from build123d import *

# Parameters (mm, degrees)
F1_DEPTH = 70
F3_DEPTH = 5
F4_DEPTH = 25


with BuildPart() as f1:
    # F0 (on Front) → F1 (new body)
    with BuildSketch(Plane.XZ):
        Polygon((-54.826997, 51.085521), (-62.88556, 51.085521), (-62.88556, -34.104981), (92.241742, -34.104981), (92.241742, -22.304947), (17.98786, -22.304947), (17.98786, 51.085521), (7.051241, 51.085521), (-13.095161, 5.612212), (-13.095161, -5.612212), (-22.592751, -5.612212), (-22.592751, 5.612212), align=None)
    extrude(amount=F1_DEPTH)

    # F2 (on face) → F3 (join)
    with BuildSketch(Plane.XY.offset(-22.304947)):
        with BuildLine():
            Line((77.980134, -20.254048), (34.15819, -20.254048))
            ThreePointArc((34.15819, -20.254048), (30.622656, -21.718514), (29.15819, -25.254048))
            Line((29.15819, -25.254048), (29.15819, -43.014842))
            ThreePointArc((29.15819, -43.014842), (30.622656, -46.550376), (34.15819, -48.014842))
            Line((34.15819, -48.014842), (77.980134, -48.014842))
            ThreePointArc((77.980134, -48.014842), (81.515667, -46.550376), (82.980134, -43.014842))
            Line((82.980134, -43.014842), (82.980134, -25.254048))
            ThreePointArc((82.980134, -25.254048), (81.515667, -21.718514), (77.980134, -20.254048))
        make_face()
        with BuildLine():
            ThreePointArc((31.707652, -28.936601), (33.172118, -25.401067), (36.707652, -23.936601))
            Line((36.707652, -23.936601), (70.1474, -23.936601))
            ThreePointArc((70.1474, -23.936601), (73.682934, -25.401067), (75.1474, -28.936601))
            Line((75.1474, -28.936601), (75.1474, -38.765739))
            ThreePointArc((75.1474, -38.765739), (73.682934, -42.301273), (70.1474, -43.765739))
            Line((70.1474, -43.765739), (36.707652, -43.765739))
            ThreePointArc((36.707652, -43.765739), (33.172118, -42.301273), (31.707652, -38.765739))
            Line((31.707652, -38.765739), (31.707652, -28.936601))
        make_face(mode=Mode.SUBTRACT)
    extrude(amount=F3_DEPTH)

    # F3_face (on face) → F4 (cut)
    with BuildSketch(Plane(origin=(53.427526, -33.85117, -22.304947), x_dir=(1, 0, 0), z_dir=(0, 0, 1))):
        with BuildLine():
            Line((-21.719874, 4.914569), (-21.719874, -4.914569))
            ThreePointArc((-21.719874, -4.914569), (-20.255408, -8.450103), (-16.719874, -9.914569))
            Line((-16.719874, -9.914569), (16.719874, -9.914569))
            ThreePointArc((16.719874, -9.914569), (20.255408, -8.450103), (21.719874, -4.914569))
            Line((21.719874, -4.914569), (21.719874, 4.914569))
            ThreePointArc((21.719874, 4.914569), (20.255408, 8.450103), (16.719874, 9.914569))
            Line((16.719874, 9.914569), (-16.719874, 9.914569))
            ThreePointArc((-16.719874, 9.914569), (-20.255408, 8.450103), (-21.719874, 4.914569))
        make_face()
    extrude(amount=-F4_DEPTH, mode=Mode.SUBTRACT)


solid = f1.part
The listing builds one solid part. Answer for the finished solid, in the listing's coordinates (mm). A direction names the side the tool comes from. Coordinates: 2 decimals unless noted, no trailing zeros. Write each loop counter-clockwise with the first axis right and the second up, starting at its lowest first coordinate (ties: lowest second). Pieces come first, ordered by that corner, then holes. Notation, with made-up numbers: M -36.75,12.25 L 9.25,12.25 A17 ccw 9.25,20.25 Z; hole C 19,18 d2. An arc over 180 degrees is marked long. Put each result on its own line as item: value. Start each with the question number.
1. A cutting plane is placed at D-D on y = -6. Write down the section's boundary in (x, z).
2. Consider line 1 (Y direction, x = 46.5, z = -20); line 2 (X direction, y = -14, z = 2); line 3 (X direction, y = -60.5, z = -20.5). Determine where each line is inside the solid, lowest interval first. Write a range as from..to.
3. Which of the six approach directions +Z, -Z, +X, -X, +Y, -Y give full straight-line access (tool end or side, diameter ignored) to faces 1 (the flat face through (31.708, -34, -26)), 2 (the cylindrical face through (30.58, -46.51, -19.84)), 3 (the flat face through (-18, -35, -5.612)), 4 (the cylindrical face through (81.554, -21.758, -19.84))?
4. For a pull along Y with two mould halves and no side action, classify faces 5 (the flat face through (17.988, -35, 14)), 6 (the cylindrical face through (33.211, -25.362, -25.587)), 7 (the flat face through (-4, -70, 0)) as pulls with the +Y half, pulls with the -Y half, needs draft (parallel to the pull), parting line crosses it, or undercut.
5. A cutting plane is placed at B-B on y = -33. Write down the section's boundary in (x, z), then the cut area to 3 significant figures.
6. Flat-ended cylindrical pins translate along their axes: P1, Ø4, axis at x = -17, y = -19, coming from the +Z side; P2, Ø1.5, axis at y = -12.5, z = 5.5, coming from the +X side; P3, Ø10, axis at x = 37.5, y = -61.5, coming from the +Z side; P4, Ø1.5, axis at x = -27.5, z = 14.5, coming from the -Y side. Find the tip coordinate at first contact, or state that the pin passes through.
7. A cutting plane is placed at C-C on z = 12. Write down the section's boundary in (x, y), then the cut area to 3 significant figures.
8. A cutting plane is placed at A-A on x = 61.5. Write down the section's boundary in (y, z), then the cut area to 3 significant figures.
Resolved:
1. outline: M -62.89,-34.1 L 92.24,-34.1 L 92.24,-22.3 L 17.99,-22.3 L 17.99,51.09 L 7.05,51.09 L -13.1,5.61 L -13.1,-5.61 L -22.59,-5.61 L -22.59,5.61 L -54.83,51.09 L -62.89,51.09 Z
2. line 1: y = -48.01..-43.77, -23.94..-20.25
2. line 2: x = -62.89..-22.59, -13.1..17.99
2. line 3: x = -62.89..17.99
3. face 1: +Z, -Z
3. face 2: +Z, -Y
3. face 3: +Z, +Y, -Y
3. face 4: +Z, +X, +Y
4. face 5: needs draft
4. face 6: undercut
4. face 7: pulls with the -Y half
5. outline: M -62.89,-34.1 L 31.71,-34.1 L 31.71,-17.3 L 29.16,-17.3 L 29.16,-22.3 L 17.99,-22.3 L 17.99,51.09 L 7.05,51.09 L -13.1,5.61 L -13.1,-5.61 L -22.59,-5.61 L -22.59,5.61 L -54.83,51.09 L -62.89,51.09 Z; M 75.15,-34.1 L 92.24,-34.1 L 92.24,-22.3 L 82.98,-22.3 L 82.98,-17.3 L 75.15,-17.3 Z
5. area: 5,580 mm2
6. P1: stops at z = -5.61
6. P2: stops at x = 17.99
6. P3: stops at z = -22.3
6. P4: passes through
7. outline: M -62.89,-70 L -27.12,-70 L -27.12,0 L -62.89,0 Z; M -10.27,-70 L 17.99,-70 L 17.99,0 L -10.27,0 Z
7. area: 4,480 mm2
8. outline: M -70,-34.1 L -43.77,-34.1 L -43.77,-17.3 L -48.01,-17.3 L -48.01,-22.3 L -70,-22.3 Z; M -23.94,-34.1 L 0,-34.1 L 0,-22.3 L -20.25,-22.3 L -20.25,-17.3 L -23.94,-17.3 Z
8. area: 632 mm2
